Source: three-view drawing plus pictorial views. Frame: mm from the lowest corner of the part. A direction names the side the tool comes from. Round coordinates to 2 decimals unless told otherwise and drop trailing zeros. Loops run counter-clockwise (first coordinate to the right, second up) from the corner with the lowest first, then second, coordinate; pieces in that order, holes last. Notation, with made-up numbers: (66.25, -18.75) -> (102.25, -18.75) arc R13 cw to (102.25, 0.25) -> close; hole circle Ø2 at (77.25, 72). An arc over 180 degrees is marked (long way). Put each result on its own line as item: value. Start each with the question number.
1. Cut plane A-A (y = 22.5). Return the cut outline in (x, z).
2. Contact query for flat-ended pins moving along their axis: pin 1 (5 mm diameter, centred on x = 10.5, z = 6, fed in from -Y); pin 2 (7 mm diameter, centred on x = 37.66, y = 13.75, fed in from +Z); pin 3 (6 mm diameter, centred on y = 28, z = 8.5, fed in from -X); pin 4 (4 mm diameter, centred on y = 14.5, z = 9, fed in from +X) (1 decimal). Output: stop coordinate, or through.
3. Set-up query: the marked faces 5 and 6. Return all of +Z, -Z, +X, -X, +Y, -Y with unobstructed straight access to the full face (end or side cutting, diameter ignored); none if empty.
4. Cut plane C-C (y = 13.75). Return the cut outline in (x, z) (1 decimal).
5. Cut plane B-B (x = 22.5). Return the cut outline in (y, z).
6. Cut plane D-D (z = 3.5). State how many separate pieces and enclosed holes the cut face has.
7. Draft query along X for the marked faces 1, 2, 3 and 4. Return one class per face: pulls with the +X half, pulls with the -X half, needs draft (parallel to the pull), parting line crosses it, or undercut.
8. Material intervals for L1, parallel to X at y = 13.75, z = 6.5 (1 decimal); L2, parallel to Y at x = 38, z = 4.5; L3, parallel to X at y = 30, z = 8.5 (1 decimal), sorted ascending.
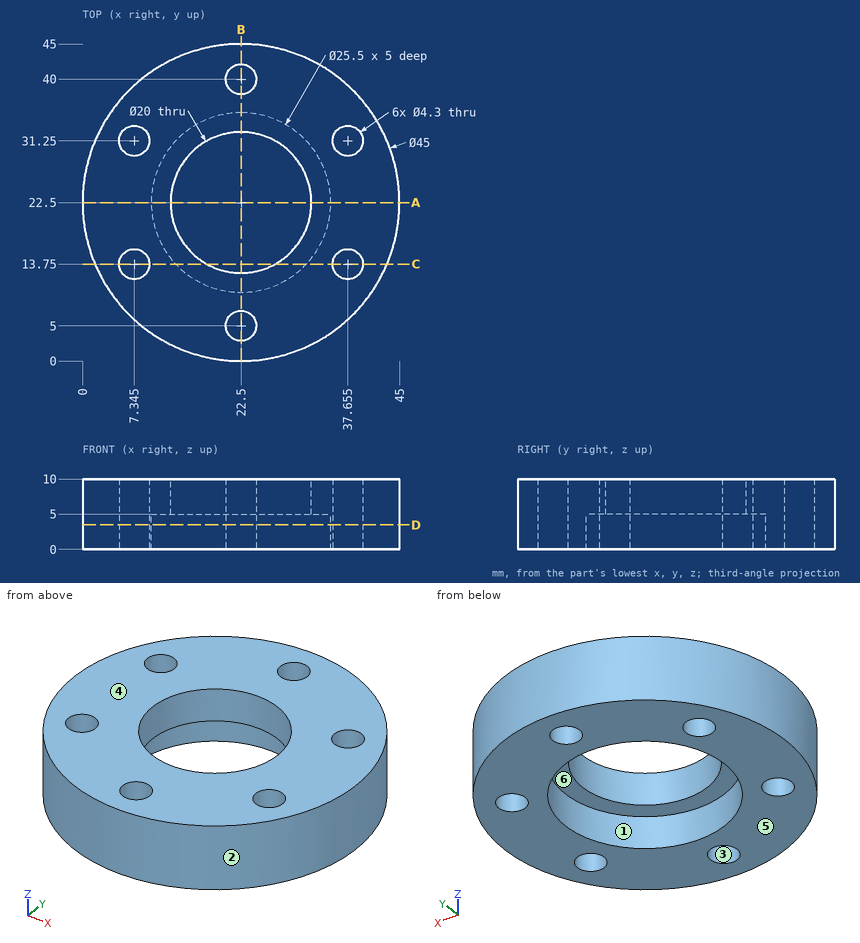
Solution:
1. outline: (0, 0) -> (9.75, 0) -> (9.75, 5) -> (12.5, 5) -> (12.5, 10) -> (0, 10) -> close; (32.5, 5) -> (35.25, 5) -> (35.25, 0) -> (45, 0) -> (45, 10) -> (32.5, 10) -> close
2. pin 1: stops at y = 2.1
2. pin 2: stops at z = 10
2. pin 3: stops at x = 0.14
2. pin 4: stops at x = 44.2
3. face 5: -Z, +X, -X, +Y, -Y
3. face 6: -Z
4. outline: (1.8, 0) -> (5.2, 0) -> (5.2, 10) -> (1.8, 10) -> close; (9.5, 0) -> (13.2, 0) -> (13.2, 5) -> (17.7, 5) -> (17.7, 10) -> (9.5, 10) -> close; (27.3, 5) -> (31.8, 5) -> (31.8, 0) -> (35.5, 0) -> (35.5, 10) -> (27.3, 10) -> close; (39.8, 0) -> (43.2, 0) -> (43.2, 10) -> (39.8, 10) -> close
5. outline: (0, 0) -> (2.85, 0) -> (2.85, 10) -> (0, 10) -> close; (7.15, 0) -> (9.75, 0) -> (9.75, 5) -> (12.5, 5) -> (12.5, 10) -> (7.15, 10) -> close; (32.5, 5) -> (35.25, 5) -> (35.25, 0) -> (37.85, 0) -> (37.85, 10) -> (32.5, 10) -> close; (42.15, 0) -> (45, 0) -> (45, 10) -> (42.15, 10) -> close
6. separate pieces: 1
6. enclosed holes: 7
7. face 1: undercut
7. face 2: parting line crosses it
7. face 3: undercut
7. face 4: needs draft
8. L1: x = 1.8 to 5.2, 9.5 to 17.7, 27.3 to 35.5, 39.8 to 43.2
8. L2: y = 6.19 to 11.63, 15.87 to 29.13, 33.37 to 38.81
8. L3: x = 1.3 to 5.6, 9.1 to 15.9, 29.1 to 35.9, 39.4 to 43.7
